Check sheet for the modelled part. Datum: model origin and axes. Units: mm. A direction names the side the tool comes from. Coordinates: 2 decimals unless noted, no trailing zeros. Order: outer loops, then holes, each group sorted by start corner. A loop starts at its lowest first (then second) coordinate and runs counter-clockwise, first axis right, second up.
from build123d import *

# Parameters (mm, degrees)
F0_W           = 50
F0_H           = 3
F1_DEPTH       = 12
F3_DEPTH       = 45
F5_DEPTH       = 120.001
F6_R           = 12
F6_R_2         = 1.65
F7_DEPTH       = 25
F9_D           = 4.1000000042
F9_CSINK_D     = 7.7978
F9_CSINK_ANGLE = 82
F10_W          = 1
F10_H          = 5
F11_DEPTH      = 0.4
F13_END_RADIUS = 35
F13_REACH      = 75.7248075794
F14_END_RADIUS = 35
F14_REACH      = 75.7248075794
F15_DEPTH      = 25


with BuildPart() as f1:
    # F0 (on Front) → F1 (new body)
    with BuildSketch(Plane.XZ):
        with BuildLine():
            Line((22.8227958083, 19.723181963), (-27.1772041917, 19.723181963))
            ThreePointArc((-27.1772041917, 19.723181963), (-37.4284668502, -5.0255553786), (-62.1772041917, -15.276818037))
            Line((-62.1772041917, -15.276818037), (-62.1772041917, -29.276818037))
            Line((-62.1772041917, -29.276818037), (57.8227958083, -29.276818037))
            Line((57.8227958083, -29.276818037), (57.8227958083, -15.276818037))
            ThreePointArc((57.8227958083, -15.276818037), (33.0740584668, -5.0255553786), (22.8227958083, 19.723181963))
        make_face()
        with Locations((-2.1772041917, 21.223181963)):
            Rectangle(F0_W, F0_H)
    extrude(amount=F1_DEPTH)

    # F2 (on face) → F3 (join)
    with BuildSketch(Plane.XZ.offset(12)):
        with BuildLine():
            Line((-25.1772041917, 19.723181963), (-27.1772041917, 19.723181963))
            ThreePointArc((-27.1772041917, 19.723181963), (-37.4284668502, -5.0255553786), (-62.1772041917, -15.276818037))
            Line((-62.1772041917, -15.276818037), (-62.1772041917, -29.276818037))
            Line((-62.1772041917, -29.276818037), (-60.1772041917, -29.276818037))
            Line((-60.1772041917, -29.276818037), (-60.1772041917, -17.2227244409))
            ThreePointArc((-60.1772041917, -17.2227244409), (-35.3164521546, -5.722839337), (-25.1772041917, 19.723181963))
        make_face()
        Polygon((-27.1772041917, 22.723181963), (-27.1772041917, 19.723181963), (-25.1772041917, 19.723181963), (20.8227958083, 19.723181963), (22.8227958083, 19.723181963), (22.8227958083, 22.723181963), align=None)
        with BuildLine():
            Line((22.8227958083, 19.723181963), (20.8227958083, 19.723181963))
            ThreePointArc((20.8227958083, 19.723181963), (30.9620437712, -5.722839337), (55.8227958083, -17.2227244409))
            Line((55.8227958083, -17.2227244409), (55.8227958083, -29.276818037))
            Line((55.8227958083, -29.276818037), (57.8227958083, -29.276818037))
            Line((57.8227958083, -29.276818037), (57.8227958083, -15.276818037))
            ThreePointArc((57.8227958083, -15.276818037), (33.0740584668, -5.0255553786), (22.8227958083, 19.723181963))
        make_face()
    extrude(amount=F3_DEPTH)

    # F4 (on face) → F5 (cut, through all)
    with BuildSketch(Plane(origin=(-62.1772041917, 0, 0), x_dir=(0, -1, 0), z_dir=(-1, 0, 0))):
        with BuildLine():
            Line((57, -15.276818037), (57, 19.723181963))
            ThreePointArc((57, 19.723181963), (26.3280584166, 2.7280262742), (12, -29.276818037))
            Line((12, -29.276818037), (57, -29.276818037))
            Line((57, -29.276818037), (57, -15.276818037))
        make_face()
    extrude(amount=-F5_DEPTH, mode=Mode.SUBTRACT)

    # F6 (on face) → F7 (cut)
    with BuildSketch(Plane.XY.offset(22.723181963)):
        with Locations((-2.1772041917, -35.85)):
            Circle(F6_R)
        with Locations((-17.6772041917, -51.35)):
            Circle(F6_R_2)
        with Locations((-17.6772041917, -20.35)):
            Circle(F6_R_2)
        with Locations((13.3227958083, -51.35)):
            Circle(F6_R_2)
        with Locations((13.3227958083, -20.35)):
            Circle(F6_R_2)
    extrude(amount=-F7_DEPTH, mode=Mode.SUBTRACT)

    # F9 (through all)
    with Locations(Plane.XZ.offset(12)):
        with Locations((-30.1772041917, -23.2497712389), (25.8227958083, -23.2497712389)):
            CounterSinkHole(F9_D / 2, F9_CSINK_D / 2, counter_sink_angle=F9_CSINK_ANGLE)

    # F10 (on face) → F11 (join)
    with BuildSketch(Plane.XY.offset(22.723181963)):
        with Locations((-2.1772041917, -2.5)):
            Rectangle(F10_W, F10_H)
    extrude(amount=F11_DEPTH)

    f13_end = (Plane(origin=(-62.1772041917, -28.5, 19.723181963), x_dir=(0, 0, 1), z_dir=(0, 1, 0)) * Cylinder(F13_END_RADIUS, 437.0700631752, mode=Mode.PRIVATE)).faces().sort_by_distance((-37.4284668502, -0.7549172174, -5.0255553786))[0]
    # F12 (on face) → F13 (join, up to the whole of a round face its end follows)
    with BuildSketch(Plane(origin=(0, 0, -29.276818037), x_dir=(1, 0, 0), z_dir=(0, 0, -1))):
        with BuildLine():
            Line((-62.1772041917, 24), (-62.1772041917, 12))
            Line((-62.1772041917, 12), (-60.1772041917, 12))
            Line((-60.1772041917, 12), (-56.2272041917, 12))
            ThreePointArc((-56.2272041917, 12), (-52.1772041917, 16.05), (-48.1272041917, 12))
            Line((-48.1272041917, 12), (-42.1772041917, 12))
            Line((-42.1772041917, 12), (-42.1772041917, 24))
            Line((-42.1772041917, 24), (-62.1772041917, 24))
        make_face()
        with BuildLine():
            Line((-56.2272041917, 12), (-48.1272041917, 12))
            ThreePointArc((-48.1272041917, 12), (-52.1772041917, 16.05), (-56.2272041917, 12))
        make_face()
    f13_long = extrude(amount=-F13_REACH, mode=Mode.PRIVATE)
    add(split(f13_long, bisect_by=f13_end, keep=Keep.TOP, mode=Mode.PRIVATE))

    f14_end = (Plane(origin=(57.8227958083, -28.5, 19.723181963), x_dir=(0, 0, 1), z_dir=(0, 1, 0)) * Cylinder(F14_END_RADIUS, 437.0700631752, mode=Mode.PRIVATE)).faces().sort_by_distance((33.0740584668, -0.7549172174, -5.0255553786))[0]
    # F12 (on face) → F14 (join, up to the whole of a round face its end follows)
    with BuildSketch(Plane(origin=(0, 0, -29.276818037), x_dir=(1, 0, 0), z_dir=(0, 0, -1))):
        with BuildLine():
            Line((37.8227958083, 24), (37.8227958083, 12))
            Line((37.8227958083, 12), (43.7727958083, 12))
            ThreePointArc((43.7727958083, 12), (47.8227958083, 16.05), (51.8727958083, 12))
            Line((51.8727958083, 12), (55.8227958083, 12))
            Line((55.8227958083, 12), (57.8227958083, 12))
            Line((57.8227958083, 12), (57.8227958083, 24))
            Line((57.8227958083, 24), (37.8227958083, 24))
        make_face()
        with BuildLine():
            Line((51.8727958083, 12), (43.7727958083, 12))
            ThreePointArc((43.7727958083, 12), (47.8227958083, 7.95), (51.8727958083, 12))
        make_face()
    f14_long = extrude(amount=-F14_REACH, mode=Mode.PRIVATE)
    add(split(f14_long, bisect_by=f14_end, keep=Keep.TOP, mode=Mode.PRIVATE))

    # F12 (on face) → F15 (cut)
    with BuildSketch(Plane(origin=(0, 0, -29.276818037), x_dir=(1, 0, 0), z_dir=(0, 0, -1))):
        with BuildLine():
            Line((-56.2272041917, 12), (-48.1272041917, 12))
            ThreePointArc((-48.1272041917, 12), (-52.1772041917, 16.05), (-56.2272041917, 12))
        make_face()
        with BuildLine():
            ThreePointArc((-56.2272041917, 12), (-52.1772041917, 7.95), (-48.1272041917, 12))
            Line((-48.1272041917, 12), (-56.2272041917, 12))
        make_face()
        with BuildLine():
            Line((51.8727958083, 12), (43.7727958083, 12))
            ThreePointArc((43.7727958083, 12), (47.8227958083, 7.95), (51.8727958083, 12))
        make_face()
        with BuildLine():
            ThreePointArc((51.8727958083, 12), (47.8227958083, 16.05), (43.7727958083, 12))
            Line((43.7727958083, 12), (51.8727958083, 12))
        make_face()
    extrude(amount=-F15_DEPTH, mode=Mode.SUBTRACT)


solid = f1.part
(1) Cross-section at D-D (y = -3.5). Enter the section's corners in (x, z), and give its area (3 significant figures).
Filled in:
outline: (-62.18, -29.28) - (57.82, -29.28) - (57.82, -15.28) arc R35 cw to (22.82, 19.72) - (22.82, 22.72) - (-1.68, 22.72) - (-1.68, 23.12) - (-2.68, 23.12) - (-2.68, 22.72) - (-27.18, 22.72) - (-27.18, 19.72) arc R35 cw to (-62.18, -15.28) - close; hole circle Ø4.1 at (-30.18, -23.25); hole circle Ø4.1 at (25.82, -23.25)
area: 4,080 mm2
(2) Tool access check on faces 4 (the flat face through (-27.177, -28, 21)), 5 (the flat face through (-3, -12, -4)), 6 (the flat face through (22.823, -28, 21)). Record the directions out of +Z, -Z, +X, -X, +Y, -Y that give a thin tool (end or side, any length) a straight path to the whole face; none if there is none.
Filled in:
face 4: +Z, -X, +Y, -Y
face 5: -Z, -Y
face 6: +Z, +X, +Y, -Y
(3) Cross-section at C-C (x = -23). Enter the section's corners in (y, z), and give its area (3 significant figures).
Filled in:
outline: (-57, 19.72) - (-12, 19.72) - (-12, -29.28) - (0, -29.28) - (0, 22.72) - (-57, 22.72) - close
area: 759 mm2
(4) Cross-section at B-B (x = 45.5). Enter the section's corners in (y, z).
Filled in:
outline: (-24, -29.28) - (-15.32, -29.28) - (-15.32, -13.04) - (-24, -13.04) - close; (-8.68, -29.28) - (0, -29.28) - (0, -13.04) - (-8.68, -13.04) - close
(5) Go/stop test with flat-tipped pins: P1, Ø2.5, axis at y = -40, z = 22, coming from the +X side; P2, Ø5.5, axis at x = -17.68, y = -51.35, coming from the +Z side; P3, Ø6, axis at x = -10.5, z = 12, coming from the -Y side. Record where each tip stops, or that it passes through.
Filled in:
P1: stops at x = 22.82
P2: stops at z = 22.72
P3: stops at y = -12
(6) Cross-section at A-A (y = -27). Enter the section's corners in (x, z).
Filled in:
outline: (-31.19, 3.45) - (-28.95, 3.45) arc R37 ccw to (-25.18, 19.72) - (-10.28, 19.72) - (-10.28, 22.72) - (-27.18, 22.72) - (-27.18, 19.72) arc R35 cw to start; (5.93, 19.72) - (20.82, 19.72) arc R37 ccw to (24.6, 3.45) - (26.84, 3.45) arc R35 cw to (22.82, 19.72) - (22.82, 22.72) - (5.93, 22.72) - close
(7) Release check for a two-part mould opening along Z. For faces 1 (the cylindrical face through (-28.67, -4.87, -21.86)), 2 (the flat face through (-3, 0, -9)), 3 (the flat face through (-16, -10, -29.277)) record: +Z half, -Z half, draft (parallel to the pull), parting line (faces both ways), or undercut.
Filled in:
face 1: undercut
face 2: draft
face 3: -Z half
(8) Thickness scan on probe 1 along X at (y, z) = (-19, -20); probe 2 along Y at (x, z) = (-22.5, 11); probe 3 along Z at (x, y) = (-7, -9). Record the ranges inside material, lowest first.
Filled in:
probe 1: x = -62.18 to -42.18, 37.82 to 57.82
probe 2: y = -12 to 0
probe 3: z = -29.28 to 22.72
